```python
from build123d import *

# Parameters (mm, degrees)
SKETCH_1_W        = 420
SKETCH_1_H        = 360
EXTRUDE_1_DEPTH   = 3
SKETCH_2_W        = 420
SKETCH_2_H        = 360
SKETCH_2_W_2      = 414
SKETCH_2_H_2      = 354
EXTRUDE_1_2_DEPTH = 477
SKETCH_3_W        = 450
SKETCH_3_H        = 530
EXTRUDE_2_DEPTH   = 3


with BuildPart() as part:
    # 草图1 → Extrude 1 (new body)
    with BuildSketch(Plane(origin=(0, 0, 0), x_dir=(1, 0, 0), z_dir=(0, 1, 0))):
        Rectangle(SKETCH_1_W, SKETCH_1_H)
    extrude(amount=EXTRUDE_1_DEPTH)

    # 草图2 → Extrude 1 2 (add)
    with BuildSketch(Plane(origin=(0, 3, 0), x_dir=(1, 0, 0), z_dir=(0, 1, 0))):
        Rectangle(SKETCH_2_W, SKETCH_2_H)
        Rectangle(SKETCH_2_W_2, SKETCH_2_H_2, mode=Mode.SUBTRACT)
    extrude(amount=EXTRUDE_1_2_DEPTH)

    # 草图3 → 凸台-拉伸2 (add)
    with BuildSketch(Plane.XY.offset(180)):
        with Locations((-5, 245)):
            Rectangle(SKETCH_3_W, SKETCH_3_H)
    extrude(amount=-EXTRUDE_2_DEPTH)


solid = part.part
```
Work out the finished part from the listing and answer in its coordinate system (mm). A direction names the side the tool comes from. Give positions to 0.01 mm unless a question says otherwise; leave off trailing zeros. Loops run counter-clockwise (first coordinate to the right, second up) from the corner with the lowest first, then second, coordinate; pieces in that order, holes last. Notation, with made-up numbers: (10.5, -28.75) -> (36.5, -28.75) arc R35 cw to (36.5, 4.25) -> close; hole circle Ø8 at (-13, 31). An arc over 180 degrees is marked (long way). One line per question, with ' | ' between items. Start each with the question number.
1) Section C-C, the plane z = 145 is taken. Determine the outline of the cut face in (x, y), then the cut area to 3 significant figures.
2) Section B-B, the plane x = -94 is taken. Determine the outline of the cut face in (y, z), then the cut area to 3 significant figures.
3) Section A-A, the plane y = 309 is taken. Determine the outline of the cut face in (x, z).
4) Each of these flat-tipped pins is pushed along its axis until it touches: pin 1 (12 mm diameter, centred on x = 130.5, z = 22.5, fed in from -Y); pin 2 (4 mm diameter, centred on y = 138.5, z = 74, fed in from +X); pin 3 (6 mm diameter, centred on x = 72.5, z = -90, fed in from +Y). Where does it stop, or does it pass through?
5) For faces 4 (the face through (-3, 238, -177)), 5 (the face through (-210, 237, 1)), 6 (the face through (-3, 0, -4)), determine the directions among +Z, -Z, +X, -X, +Y, -Y from which every point of the face is accessible in a straight line to the end or side of a thin tool.
6) Determine the mould class of faces 1 (the face through (-207, 238, 2)), 2 (the face through (-8, 249, 180)), 3 (the face through (210, 237, 1)) for opening direction X: +X half, -X half, draft (parallel to the pull), parting line (faces both ways), or undercut.
7) Straight lines are drawn through the part: L1, parallel to Z at x = -59.5, y = 19; L2, parallel to X at y = 58.5, z = -34; L3, parallel to Y at x = 53.5, z = -80.5. For each, find the intervals that lie inside material, in ascending order.
Resolved:
1) outline: (-210, 0) -> (210, 0) -> (210, 480) -> (207, 480) -> (207, 3) -> (-207, 3) -> (-207, 480) -> (-210, 480) -> close | area: 4,120 mm2
2) outline: (-20, 177) -> (0, 177) -> (0, -180) -> (480, -180) -> (480, -177) -> (3, -177) -> (3, 177) -> (510, 177) -> (510, 180) -> (-20, 180) -> close | area: 4,090 mm2
3) outline: (-230, 177) -> (-210, 177) -> (-210, -180) -> (210, -180) -> (210, 177) -> (220, 177) -> (220, 180) -> (-230, 180) -> close; hole (-207, -177) -> (207, -177) -> (207, 177) -> (-207, 177) -> close
4) pin 1: y = 0 | pin 2: x = 210 | pin 3: y = 3
5) face 4: +Y | face 5: -Z, -X, +Y, -Y | face 6: -Z, +X, -X, -Y
6) face 1: undercut | face 2: draft | face 3: +X half
7) L1: -180 to -177, 177 to 180 | L2: -210 to -207, 207 to 210 | L3: 0 to 3
